Part model, mm, in its own coordinate system. A direction names the side the tool comes from. Coordinates: 2 decimals unless noted, no trailing zeros. Loops run counter-clockwise (first coordinate to the right, second up) from the corner with the lowest first, then second, coordinate; pieces in that order, holes last. Notation, with made-up numbers: (13.5, -1.75) -> (52.5, -1.75) arc R25 ccw to (52.5, 35.25) -> close; hole circle Ø8 at (-1, 75). An arc over 180 degrees is marked (long way). One line per question, with ' | ' between items. Start each with the question number.
1) Cut at D-D (y = 65). List the corners of the cut face in (x, z), plus the area to 3 significant figures.
2) Drop flat-ended pins along their axis: pin 1 (1.2 mm diameter, centred on x = 3, z = 19, fed in from +Y); pin 2 (4 mm diameter, centred on y = 10.6, z = 120.88, fed in from -X); pin 3 (2 mm diameter, centred on x = 2.5, y = 87, fed in from +Z); pin 4 (6.5 mm diameter, centred on y = 25, z = 150.75, fed in from -X). Give the stop position or say it passes through.
3) Probe L1, parallel to Y at x = 1.4, z = 25.5; L2, parallel to Y at x = 3.05, z = 150.75 (3 decimals); L3, parallel to Z at x = 3.3, y = 9. List the from-to ranges inside material, lowest first. Write a range as from..to.
4) Cut at C-C (z = 150.75). List the corners of the cut face in (x, y) (3 decimals).
5) Cut at B-B (y = 29.5). List the corners of the cut face in (x, z), plus the area to 3 significant figures.
6) 3-axis set-ups, long thin cutter, end or side, ignore diameter. For faces 1 (the face through (2, -10, 28)), 2 (the face through (2, 18, 28)), 3 (the face through (0, 27, 84)): which of +Z, -Z, +X, -X, +Y, -Y reach the whole face in a straight line?
7) Cut at A-A (x = 0.9). List the corners of the cut face in (y, z) (3 decimals).
8) Two-plate mould, pull along Z, no slides. Class faces 4 (the face through (2, 124, 85.7)), 5 (the face through (1.972, 10.711, 123.377)), 6 (the face through (1.972, 29.415, 132.16)), 7 (the face through (1.972, 4.605, 124.286)): released by +Z, released by -Z, zero draft, split by the parting line, or undercut.
from build123d import *

# Parameters (mm, degrees)
SKETCH1_R           = 2.5
SKETCH1_R_2         = 6.25
BOSS_EXTRUDE1_DEPTH = 4
SKETCH2_W           = 4
SKETCH2_H           = 28
BOSS_EXTRUDE2_DEPTH = 1.94


with BuildPart() as part:
    # Sketch1 → Boss-Extrude1 (new body)
    with BuildSketch(Plane(origin=(0, 0, 0), x_dir=(0, 0, -1), z_dir=(1, 0, 0))):
        with BuildLine():
            ThreePointArc((-57.5, 18), (-70.338674346, 23.330913022), (-75.625323458, 36.187877429))
            Line((-75.625323458, 36.187877429), (-81.75, 120))
            ThreePointArc((-81.75, 120), (-85.75, 124), (-89.75, 120))
            Line((-89.75, 120), (-115.82263113, 27.253642352))
            Line((-115.82263113, 27.253642352), (-148.961993572, 31.638422856))
            ThreePointArc((-148.961993572, 31.638422856), (-157.193398915, 27.397547793), (-153.736313474, 18.807459581))
            Line((-153.736313474, 18.807459581), (-94, -10))
            ThreePointArc((-94, -10), (-75.75, -17.559397513), (-57.5, -10))
            Line((-57.5, -10), (0, -10))
            Line((0, -10), (0, 18))
            Line((0, 18), (-57.5, 18))
        make_face()
        with Locations((-150.75, 25)):
            Circle(SKETCH1_R, mode=Mode.SUBTRACT)
        with Locations((-120.879671399, 10.600773875)):
            Circle(SKETCH1_R, mode=Mode.SUBTRACT)
        with Locations((-75.75, 0)):
            Circle(SKETCH1_R_2, mode=Mode.SUBTRACT)
        with Locations((-105.136571318, 45.63560228)):
            Circle(SKETCH1_R, mode=Mode.SUBTRACT)
        with Locations((-92.213009764, 95.208724602)):
            Circle(SKETCH1_R, mode=Mode.SUBTRACT)
        with Locations((-85.75, 120)):
            Circle(SKETCH1_R, mode=Mode.SUBTRACT)
    extrude(amount=BOSS_EXTRUDE1_DEPTH)

    # Sketch2 → Boss-Extrude2 (add)
    with BuildSketch(Plane(origin=(0, 0, 0), x_dir=(-1, 0, 0), z_dir=(0, 0, -1))):
        with Locations((-2, 4)):
            Rectangle(SKETCH2_W, SKETCH2_H)
    extrude(amount=BOSS_EXTRUDE2_DEPTH)


solid = part.part
Reported:
1) outline: (0, 77.73) -> (4, 77.73) -> (4, 105.21) -> (0, 105.21) -> close | area: 110 mm²
2) pin 1: stops at y = 18 | pin 2: passes through | pin 3: stops at z = 99.31 | pin 4: stops at x = 0
3) L1: y = -10..18 | L2: y = 17.367..22.5, 27.5..31.875 | L3: z = -1.94..118.96, 122.8..133.4
4) outline: (0, 17.367) -> (4, 17.367) -> (4, 22.5) -> (0, 22.5) -> close; (0, 27.5) -> (4, 27.5) -> (4, 31.875) -> (0, 31.875) -> close
5) outline: (0, 74.37) -> (4, 74.37) -> (4, 115.19) -> (0, 115.19) -> close; (0, 132.8) -> (4, 132.8) -> (4, 155.95) -> (0, 155.95) -> close | area: 256 mm²
6) face 1: -Z, +X, -X, -Y | face 2: -Z, +X, -X, +Y | face 3: +Z, -Z, -X, +Y, -Y
7) outline: (-10, -1.94) -> (18, -1.94) -> (18, 57.5) arc R18.125 cw to (36.188, 75.625) -> (120, 81.75) arc R4 ccw to (120, 89.75) -> (27.254, 115.823) -> (31.638, 148.962) arc R6.875 ccw to (18.807, 153.736) -> (-10, 94) arc R25.809 ccw to (-10, 57.5) -> close; hole circle Ø12.5 at (0, 75.75); hole circle Ø5 at (10.601, 120.88); hole circle Ø5 at (25, 150.75); hole circle Ø5 at (45.636, 105.137); hole circle Ø5 at (95.209, 92.213); hole circle Ø5 at (120, 85.75)
8) face 4: split by the parting line | face 5: undercut | face 6: undercut | face 7: released by +Z
